The listing builds one solid part. Answer for the finished solid, in the listing's coordinates (mm). Face numbers are marked on the shaded views. A direction names the side the tool comes from. Give positions to 0.01 mm unless a question says otherwise; leave off trailing zeros. Loops run counter-clockwise (first coordinate to the right, second up) from the corner with the lowest first, then second, coordinate; pieces in that order, holes last. Notation, with made-up numbers: M 55,-25.5 L 102,-25.5 A32 ccw 102,4.5 Z; hole C 33.25,44.25 d6. An arc over 180 degrees is marked long. Return JSON: item names as keys, results as strings.
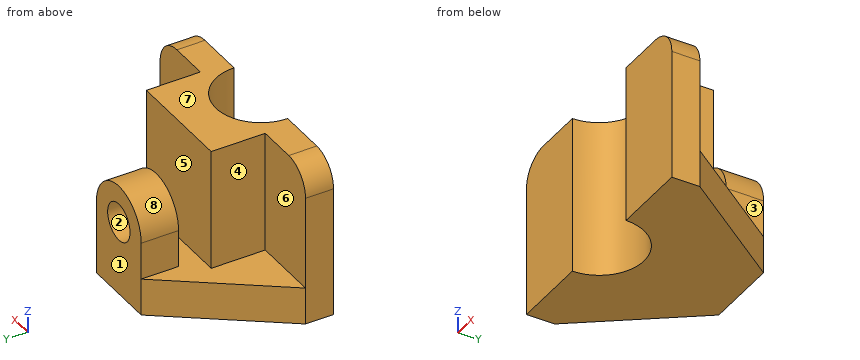
from build123d import *

# Parameters (mm, degrees)
EXTRUDE_1_DEPTH          = 85
CUT_EXTRUDE_1_DEPTH      = 116.666660236
CUT_EXTRUDE_1_DEPTH_BACK = 116.666660236
EXTRUDE_2_DEPTH          = 20
SKETCH_5_R               = 10
EXTRUDE_3_DEPTH          = 20
FILLET_1_R               = 15


with BuildPart() as part:
    # 스케치1 → 보스-돌출1 (new body)
    with BuildSketch(Plane.XY):
        Polygon((-65, 0), (65, 0), (65, 15), (29, 15), (29, 43.917835671), (-29, 43.917835671), (-29, 15), (-65, 15), align=None)
    extrude(amount=EXTRUDE_1_DEPTH)

    # 스케치2 → 컷-돌출1 (cut, two sides: drawn at the far end of the back side and taken through both)
    with BuildSketch(Plane.XY.offset(85).offset(-CUT_EXTRUDE_1_DEPTH_BACK)):
        with BuildLine():
            ThreePointArc((24, 0), (0, 24), (-24, 0))
            Line((-24, 0), (24, 0))
        make_face()
    extrude(amount=CUT_EXTRUDE_1_DEPTH + CUT_EXTRUDE_1_DEPTH_BACK, mode=Mode.SUBTRACT)

    # 스케치4 → 보스-돌출2 (add)
    with BuildSketch(Plane(origin=(0, 0, 0), x_dir=(-1, 0, 0), z_dir=(0, 0, -1))):
        Polygon((-65, 15), (-20, 76), (20, 76), (65, 15), (29, 15), (29, 43.917835671), (-29, 43.917835671), (-29, 15), align=None)
    extrude(amount=-EXTRUDE_2_DEPTH)

    # 스케치5 → 보스-돌출3 (add)
    with BuildSketch(Plane(origin=(0, 76, 0), x_dir=(1, 0, 0), z_dir=(0, 1, 0))):
        with BuildLine():
            Line((-20, 0), (-20, -40))
            ThreePointArc((-20, -40), (0, -60), (20, -40))
            Line((20, -40), (20, 0))
            Line((20, 0), (-20, 0))
        make_face()
        with Locations(Location((0, -40, 0), (0, 0, 270))):
            Circle(SKETCH_5_R, mode=Mode.SUBTRACT)
    extrude(amount=-EXTRUDE_3_DEPTH)

    # 필렛1
    fillet_1_edges = [part.edges().sort_by_distance(p)[0] for p in [
        (65, 7.5, 85),
        (-65, 7.5, 85),
    ]]
    fillet(fillet_1_edges, radius=FILLET_1_R)


solid = part.part
(1) The part is cut by section C-C (z = 66). Determine the outline of the cut face in (x, y).
Values follow:
{"outline": "M -65,0 L -24,0 A24 cw 24,0 L 65,0 L 65,15 L 29,15 L 29,43.92 L -29,43.92 L -29,15 L -65,15 Z"}
(2) The part is cut by section D-D (z = 45.5). Determine the outline of the cut face in (x, y), and give its area (3 significant figures).
Values follow:
{"outline": "M -65,0 L -24,0 A24 cw 24,0 L 65,0 L 65,15 L 29,15 L 29,43.92 L -29,43.92 L -29,15 L -65,15 Z; M -19.23,56 L -8.35,56 L -8.35,76 L -19.23,76 Z; M 8.35,56 L 19.23,56 L 19.23,76 L 8.35,76 Z", "area": "3,160 mm²"}
(3) Determine the mould class of the marked faces 1, 2, 3 and 4 for opening direction X: released by +X, released by -X, zero draft, split by the parting line, or undercut.
Values follow:
{"face 1": "zero draft", "face 2": "undercut", "face 3": "released by +X", "face 4": "released by -X"}
(4) Straight lines are drawn through the part: line 1 along X through (y, z) = (65, 40); line 2 along Y through (x, z) = (-47.5, 66.5); line 3 along X through (y, z) = (37, 39). For each, find the intervals that lie inside material, in ascending order.
Values follow:
{"line 1": "-20 to -10, 10 to 20", "line 2": "0 to 15", "line 3": "-29 to 29"}
(5) The part is cut by section A-A (x = 0). Determine the outline of the cut face in (y, z).
Values follow:
{"outline": "M 24,0 L 76,0 L 76,30 L 56,30 L 56,20 L 43.92,20 L 43.92,85 L 24,85 Z; M 56,50 L 76,50 L 76,60 L 56,60 Z"}
(6) The part is cut by section B-B (y = 10). Determine the outline of the cut face in (x, z), and give its area (3 significant figures).
Values follow:
{"outline": "M -65,0 L -21.82,0 L -21.82,85 L -50,85 A15 ccw -65,70 Z; M 21.82,0 L 65,0 L 65,70 A15 ccw 50,85 L 21.82,85 Z", "area": "7,240 mm²"}
(7) Given pin 1 (17.5 mm diameter, centred on x = 8.5, z = 44.5, fed in from +Y); pin 2 (16 mm diameter, centred on y = 70.5, z = 29.5, fed in from +X); pin 3 (2 mm diameter, centred on y = 28.5, z = 14, fed in from +X); pin 4 (12 mm diameter, centred on x = -2, y = 55.5, fed in from +Z), each flat-ended and moving along its own axis, determine where each tip first touches the part or whether it passes through.
Values follow:
{"pin 1": "y = 76", "pin 2": "x = 20", "pin 3": "x = 55.78", "pin 4": "z = 60"}
(8) A tool of negligible diameter and unlimited length cuts with its end or side. For the marked faces 5, 6, 7 and 8, from which of +Z, -Z, +X, -X, +Y, -Y can it reach the whole face along a straight path? Write none if from no direction.
Values follow:
{"face 5": "+Z, +X, -X", "face 6": "+Z, -X, +Y", "face 7": "+Z, +X, -X, +Y, -Y", "face 8": "+Z, +Y"}
